Part model, mm, in its own coordinate system. Give positions to 0.01 mm unless a question says otherwise; leave off trailing zeros. Write each loop counter-clockwise with the first axis right and the second up, starting at its lowest first coordinate (ties: lowest second). Pieces come first, ordered by that corner, then holes. Notation, with made-up numbers: M 8.5,71 L 47.5,71 A27 ccw 47.5,108 Z; hole C -20,-2.75 d11. An arc over 180 degrees is marked long. Use a Markdown table: item, result.
```python
from build123d import *

# Parameters (mm, degrees)
SKETCH1_W           = 450
SKETCH1_H           = 450
SKETCH1_R           = 4
SKETCH1_R_2         = 25
BOSS_EXTRUDE1_DEPTH = 5


with BuildPart() as part:
    # Sketch1 → Boss-Extrude1 (new, symmetric)
    with BuildSketch(Plane.XY):
        Rectangle(SKETCH1_W, SKETCH1_H)
        Circle(SKETCH1_R, mode=Mode.SUBTRACT)
        with Locations((-167.5, -167.5)):
            Circle(SKETCH1_R_2, mode=Mode.SUBTRACT)
        with Locations((167.5, -167.5)):
            Circle(SKETCH1_R_2, mode=Mode.SUBTRACT)
        with Locations((167.5, 167.5)):
            Circle(SKETCH1_R_2, mode=Mode.SUBTRACT)
        with Locations((-167.5, 167.5)):
            Circle(SKETCH1_R_2, mode=Mode.SUBTRACT)
    extrude(amount=BOSS_EXTRUDE1_DEPTH, both=True)


solid = part.part
```
1. Cut at A-A, the plane x = -167.5. Give the cut face in (y, z), then the cut area to 3 significant figures.
Findings below:
| item | result |
|---|---|
| outline | M -225,-5 L -192.5,-5 L -192.5,5 L -225,5 Z; M -142.5,-5 L 142.5,-5 L 142.5,5 L -142.5,5 Z; M 192.5,-5 L 225,-5 L 225,5 L 192.5,5 Z |
| area | 3,500 mm2 |
2. Drill centre lines: L1, parallel to Y at x = -167.5, z = 1.5; L2, parallel to Y at x = 159.5, z = -4; L3, parallel to Y at x = 0, z = 0. Where is each one in solid material? Low to high.
Findings below:
| item | result |
|---|---|
| L1 | -225 to -192.5, -142.5 to 142.5, 192.5 to 225 |
| L2 | -225 to -191.19, -143.81 to 143.81, 191.19 to 225 |
| L3 | -225 to -4, 4 to 225 |
3. Cut at C-C, the plane z = -1.25. Give the cut face in (x, y).
Findings below:
| item | result |
|---|---|
| outline | M -225,-225 L 225,-225 L 225,225 L -225,225 Z; hole C -167.5,-167.5 d50; hole C -167.5,167.5 d50; hole C 0,0 d8; hole C 167.5,-167.5 d50; hole C 167.5,167.5 d50 |
4. Two-plate mould, pull along X, no slides. Class faces 1 (the cylindrical face through (-170.755, 192.287, -0.07)), 2 (the flat face through (225, -3, 0)), 3 (the flat face through (-3, 3, -5)): released by +X, released by -X, zero draft, split by the parting line, or undercut.
Findings below:
| item | result |
|---|---|
| face 1 | undercut |
| face 2 | released by +X |
| face 3 | zero draft |
5. Drop a flat-ended pin along its axis: P1, Ø6.5, axis at x = 0, y = 0, coming from the +Z side. Give the stop position or say it passes through.
Findings below:
| item | result |
|---|---|
| P1 | through |
